from build123d import *

# Parameters (mm, degrees)
F3_T1_DEPTH = 28
F3_T3_DEPTH = 44.1725614133
F5_W        = 2.5
F5_H        = 2.5


# Not quite as in the source:
# - a fillet or chamfer that OpenCascade refuses, or shapes differently, is made with other operations: its cross-section is extruded or revolved along the edge and cut away or added
# - two fillets or chamfers of one size are made in one step


with BuildPart() as f2:
    # F2: sweep along a path in F1
    with BuildLine(Plane.XY) as f2_path:
        Line((0, 0), (0, 3))
    # F0 (on Front) → F2 (sweep)
    with BuildSketch(Plane.XZ):
        Polygon((-12, 0), (0, 0), (12, 0), (12, 12), (4, 7.8411921859), (0, 7.8411921859), (-4, 7.8411921859), (-12, 12), align=None)
    sweep(path=f2_path.line)

    # F3: fillet of radius 5 on 4 edges, made by hand

    # F3_s2 → F3_t1 (cut)
    with BuildSketch(Plane.XZ.offset(-15.5)):
        with BuildLine():
            ThreePointArc((-7, 0), (-10.5355339059, 1.4644660941), (-12, 5))
            Line((-12, 5), (-12, 0))
            Line((-12, 0), (-7, 0))
        make_face()
        with BuildLine():
            ThreePointArc((7, 0), (10.5355339059, 1.4644660941), (12, 5))
            Line((12, 5), (12, 0))
            Line((12, 0), (7, 0))
        make_face()
    extrude(amount=F3_T1_DEPTH, mode=Mode.SUBTRACT)

    # F3_s4 → F3_t3 (cut)
    with BuildSketch(Plane.XZ.offset(-23.5862807066)):
        with BuildLine():
            ThreePointArc((-4.6937567356, 8.2018423025), (-9.5950706809, 8.0393159966), (-12, 3.7654877173))
            Line((-12, 3.7654877173), (-12, 12))
            Line((-12, 12), (-4.6937567356, 8.2018423025))
        make_face()
        with BuildLine():
            ThreePointArc((4.6937567356, 8.2018423025), (9.5950706809, 8.0393159966), (12, 3.7654877173))
            Line((12, 3.7654877173), (12, 12))
            Line((12, 12), (4.6937567356, 8.2018423025))
        make_face()
    extrude(amount=F3_T3_DEPTH, mode=Mode.SUBTRACT)

    # F7: sweep along a path in F6
    with BuildLine(Plane.XZ) as f7_path:
        Line((0, -1.2934210245), (0, 11.7065789755))
    # F5 (on Top) → F7 (sweep, cut)
    with BuildSketch(Plane.XY):
        with Locations((0, 1.4747590758)):
            Rectangle(F5_W, F5_H)
    sweep(path=f7_path.line, mode=Mode.SUBTRACT)


solid = f2.part
Part model, mm, in its own coordinate system. A direction names the side the tool comes from. Coordinates: 2 decimals unless noted, no trailing zeros. Write each loop counter-clockwise with the first axis right and the second up, starting at its lowest first coordinate (ties: lowest second). Pieces come first, ordered by that corner, then holes. Notation, with made-up numbers: M -1.75,73 L 9.25,73 A28 ccw 9.25,111 Z; hole C -39,53.25 d3. An arc over 180 degrees is marked long. Return JSON: item names as keys, results as strings.
1. Saw through at B-B, the plane y = 1.1. Write the cut outline in (x, z).
Determined:
{"outline": "M -11.96,4.38 A5 ccw -7,0 L -1.25,0 L -1.25,7.84 L -4,7.84 L -4.69,8.2 A5 ccw Z; M 1.25,0 L 7,0 A5 ccw 11.96,4.38 A5 ccw 4.69,8.2 L 4,7.84 L 1.25,7.84 Z"}
2. 3-axis set-ups, long thin cutter, end or side, ignore diameter. For faces 1 (the face through (-10, 2, 1)), 2 (the face through (0, 2.725, 4)): which of +Z, -Z, +X, -X, +Y, -Y reach the whole face in a straight line?
Determined:
{"face 1": "-Z, -X, +Y, -Y", "face 2": "+Z, -Z"}
3. Saw through at C-C, the plane x = 2.5. Write the cut outline in (y, z).
Determined:
{"outline": "M 0,0 L 3,0 L 3,7.84 L 0,7.84 Z"}
4. Saw through at A-A, the plane z = 1. Write the cut outline in (x, y), then the cut area to 4 significant figures.
Determined:
{"outline": "M -10,0 L 10,0 L 10,3 L -10,3 Z; hole M -1.25,0.22 L 1.25,0.22 L 1.25,2.72 L -1.25,2.72 Z", "area": "53.75 mm²"}
5. Probe L1, parallel to Y at x = 0.75, z = 6.25; L2, parallel to X at y = 2.6, z = 3.75; L3, parallel to X at y = 1.35, z = 1.25. List the from-to ranges inside material, lowest first.
Determined:
{"L1": "0 to 0.22, 2.72 to 3", "L2": "-11.84 to -1.25, 1.25 to 11.84", "L3": "-10.31 to -1.25, 1.25 to 10.31"}
6. Pull direction Y, two halves, no side cores. Call faces 3 (the face through (0, 0, 4)), 4 (the face through (-1.25, 1, 4)), 5 (the face through (-9.27, 1.52, 8.22)): pulls with the +Y half, pulls with the -Y half, needs draft (parallel to the pull), parting line crosses it, or undercut.
Determined:
{"face 3": "pulls with the -Y half", "face 4": "undercut", "face 5": "needs draft"}
7. Saw through at D-D, the plane z = 3.5. Write the cut outline in (x, y), then the cut area to 3 significant figures.
Determined:
{"outline": "M -11.77,0 L 11.77,0 L 11.77,3 L -11.77,3 Z; hole M -1.25,0.22 L 1.25,0.22 L 1.25,2.72 L -1.25,2.72 Z", "area": "64.4 mm²"}
8. Flat gauge pin, fed straight in: pin 1 Ø1.5 at (x, y) = (4, 1) entering from +Z. Where does the tip first touch, or does it go through?
Determined:
{"pin 1": "z = 8.23"}
